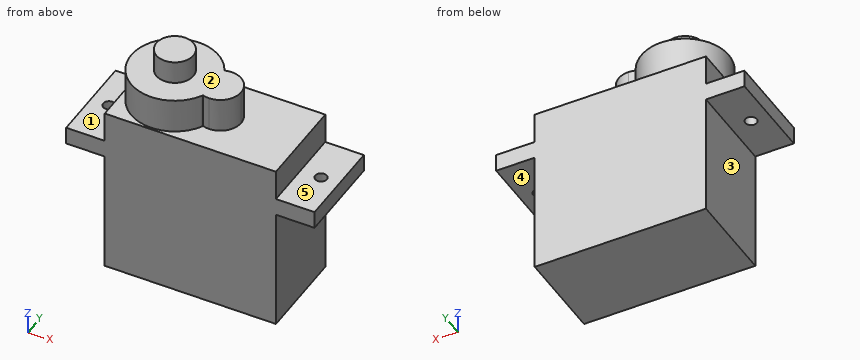
from build123d import *

# Parameters (mm, degrees)
F1_DEPTH = 11.8
F2_R     = 2.4
F3_DEPTH = 4.5
F4_DEPTH = 7.5
F2_R_2   = 0.75
F5_DEPTH = 22.301


with BuildPart() as f1:
    # F0 (on Front) → F1 (new body)
    with BuildSketch(Plane.XZ):
        Polygon((5, 16), (5, 0), (27.2, 0), (27.2, 16), (32.2, 16), (32.2, 18.3), (27.2, 18.3), (27.2, 22.3), (5, 22.3), (5, 18.3), (0, 18.3), (0, 16), align=None)
    extrude(amount=F1_DEPTH)

    # F2 (on face) → F3 (join)
    with BuildSketch(Plane.XY.offset(22.3)):
        with BuildLine():
            ThreePointArc((16.55, -5.9), (16.3947418047, -4.5845865669), (15.9375, -3.3414664845))
            ThreePointArc((15.9375, -3.3414664845), (14.1, -5.9), (15.9375, -8.4585335155))
            ThreePointArc((15.9375, -8.4585335155), (16.3947418047, -7.2154134331), (16.55, -5.9))
        make_face()
        with BuildLine():
            ThreePointArc((15.9375, -3.3414664845), (15.9008072344, -3.2704701932), (15.8631139419, -3.2))
            ThreePointArc((15.8631139419, -3.2), (5.25, -5.9), (15.8631139419, -8.6))
            ThreePointArc((15.8631139419, -8.6), (15.9008072344, -8.5295298068), (15.9375, -8.4585335155))
            ThreePointArc((15.9375, -8.4585335155), (14.1, -5.9), (15.9375, -3.3414664845))
        make_face()
        with Locations((10.9, -5.9)):
            Circle(F2_R, mode=Mode.SUBTRACT)
        with BuildLine():
            ThreePointArc((16.8, -3.2), (16.3629876958, -3.235601335), (15.9375, -3.3414664845))
            ThreePointArc((15.9375, -3.3414664845), (16.3947418047, -4.5845865669), (16.55, -5.9))
            ThreePointArc((16.55, -5.9), (16.3947418047, -7.2154134331), (15.9375, -8.4585335155))
            ThreePointArc((15.9375, -8.4585335155), (16.3629876958, -8.564398665), (16.8, -8.6))
            ThreePointArc((16.8, -8.6), (18.7091883092, -7.8091883092), (19.5, -5.9))
            ThreePointArc((19.5, -5.9), (18.7091883092, -3.9908116908), (16.8, -3.2))
        make_face()
    extrude(amount=F3_DEPTH)

    # F4 (add): a face of the model
    f4_faces = [f1.faces().sort_by_distance(p)[0] for p in [
        (10.9, -5.9, 22.3),
    ]]
    extrude(f4_faces, amount=F4_DEPTH)

    # F2 (on face) → F5 (cut, through all)
    with BuildSketch(Plane.XY.offset(22.3)):
        with Locations((2.35, -5.9)):
            Circle(F2_R_2)
        with Locations((29.85, -5.9)):
            Circle(F2_R_2)
    extrude(amount=-F5_DEPTH, mode=Mode.SUBTRACT)


solid = f1.part
Check sheet for the modelled part. Datum: model origin and axes. Units: mm. Face numbers are marked on the shaded views. A direction names the side the tool comes from. Round coordinates to 2 decimals unless told otherwise and drop trailing zeros. Order: outer loops, then holes, each group sorted by start corner. A loop starts at its lowest first (then second) coordinate and runs counter-clockwise, first axis right, second up.
Q1. Set-up check for the marked faces 1, 2, 3, 4 and 5: record each of +Z, -Z, +X, -X, +Y, -Y from which the full face is reachable in a straight line by a thin tool's end or side.
Filled sheet:
face 1: +Z, -X, +Y, -Y
face 2: +Z
face 3: -Z, -X, +Y, -Y
face 4: -Z, +X, +Y, -Y
face 5: +Z, +X, +Y, -Y
Q2. Cross-section at C-C, the plane y = -9.75. Enter the section's corners in (x, z).
Filled sheet:
outline: (0, 16) - (5, 16) - (5, 0) - (27.2, 0) - (27.2, 16) - (32.2, 16) - (32.2, 18.3) - (27.2, 18.3) - (27.2, 22.3) - (15.04, 22.3) - (15.04, 26.8) - (6.76, 26.8) - (6.76, 22.3) - (5, 22.3) - (5, 18.3) - (0, 18.3) - close
Q3. Cross-section at D-D, the plane z = 19. Enter the section's corners in (x, y).
Filled sheet:
outline: (5, -11.8) - (27.2, -11.8) - (27.2, 0) - (5, 0) - close
Q4. Cross-section at B-B, the plane x = 10.9. Enter the section's corners in (y, z).
Filled sheet:
outline: (-11.8, 0) - (0, 0) - (0, 22.3) - (-0.25, 22.3) - (-0.25, 26.8) - (-3.5, 26.8) - (-3.5, 29.8) - (-8.3, 29.8) - (-8.3, 26.8) - (-11.55, 26.8) - (-11.55, 22.3) - (-11.8, 22.3) - close
Q5. Depth check by flat-ended pin: P1, Ø1, axis at y = -1.5, z = 5, coming from the -X side; P2, Ø5.5, axis at x = 3, y = -3.5, coming from the +Z side; P3, Ø3, axis at y = -5, z = 20, coming from the +X side; P4, Ø0.9, axis at x = 2.35, y = -5.9, coming from the -Z side. Enter the tip coordinate at first touch or a pass-through.
Filled sheet:
P1: stops at x = 5
P2: stops at z = 26.8
P3: stops at x = 27.2
P4: passes through
Q6. Scan lines: L1, parallel to Y at x = 2.35, z = 17.5; L2, parallel to X at y = -5.75, z = 16.5; L3, parallel to X at y = -9.5, z = 18.75. Record each from-to range of solid material in increasing order.
Filled sheet:
L1: y = -11.8 to -6.65, -5.15 to 0
L2: x = 0 to 1.62, 3.08 to 29.12, 30.58 to 32.2
L3: x = 5 to 27.2
Q7. Cross-section at A-A, the plane x = 2.35. Enter the section's corners in (y, z).
Filled sheet:
outline: (-11.8, 16) - (-6.65, 16) - (-6.65, 18.3) - (-11.8, 18.3) - close; (-5.15, 16) - (0, 16) - (0, 18.3) - (-5.15, 18.3) - close
